The model under review builds one solid part; all positions refer to its coordinate system, in mm. A direction names the side the tool comes from. Give positions to 0.01 mm unless a question says otherwise; leave off trailing zeros. Loops run counter-clockwise (first coordinate to the right, second up) from the corner with the lowest first, then second, coordinate; pieces in that order, holes last. Notation, with made-up numbers: M 19,-22 L 50,-22 A11 cw 50,-3 Z; hole C 78,55.5 d3. An arc over 180 degrees is marked long. Put each result on its own line as item: value. Start each with the question number.
```python
from build123d import *

# Parameters (mm, degrees)
SKETCH1_W           = 50
SKETCH1_H           = 50
BOSS_EXTRUDE1_DEPTH = 2
SKETCH2_R           = 11
CUT_EXTRUDE1_DEPTH  = 36.411862419
CHAMFER1_SIZE       = 6
CHAMFER2_SIZE       = 6
CUT_EXTRUDE2_DEPTH  = 36.411862419
CIRPATTERN1_COUNT   = 4
SKETCH4_R           = 2
CUT_EXTRUDE3_DEPTH  = 36.411862419
SKETCH5_W           = 50
SKETCH5_H           = 2
BOSS_EXTRUDE5_DEPTH = 48
CHAMFER3_SIZE       = 6
CHAMFER4_SIZE       = 6
CUT_EXTRUDE5_DEPTH  = 74.681748079
BOSS_EXTRUDE6_START = -1
BOSS_EXTRUDE6_DEPTH = 1.000012
FILLET1_R           = 3


with BuildPart() as part:
    # Sketch1 → Boss-Extrude1 (new body)
    with BuildSketch(Plane.XY):
        Rectangle(SKETCH1_W, SKETCH1_H)
    extrude(amount=BOSS_EXTRUDE1_DEPTH)

    # Sketch2 → Cut-Extrude1 (cut, through all)
    with BuildSketch(Plane.XY.offset(2)):
        Circle(SKETCH2_R)
    extrude(amount=-CUT_EXTRUDE1_DEPTH, mode=Mode.SUBTRACT)

    # Chamfer1
    chamfer1_edges = [part.edges().sort_by_distance(p)[0] for p in [
        (-25, 25, 1),
    ]]
    chamfer(chamfer1_edges, length=CHAMFER1_SIZE)

    # Chamfer2
    chamfer2_edges = [part.edges().sort_by_distance(p)[0] for p in [
        (25, 25, 1),
    ]]
    chamfer(chamfer2_edges, length=CHAMFER2_SIZE)

    # Sketch3 → Cut-Extrude2 (cut, through all)
    with BuildSketch(Plane.XY.offset(2)):
        with BuildLine():
            Line((8.63247336, 12.016622274), (14.958263021, 16.914007818))
            ThreePointArc((14.958263021, 16.914007818), (17.764056822, 16.556906789), (17.406955793, 13.751112987))
            Line((17.406955793, 13.751112987), (11.081166132, 8.853727444))
            ThreePointArc((11.081166132, 8.853727444), (8.27537233, 9.210828473), (8.63247336, 12.016622274))
        make_face()
    cut_extrude2 = extrude(amount=-CUT_EXTRUDE2_DEPTH, mode=Mode.SUBTRACT)

    # CirPattern1: Cut-Extrude2 ×4 about axis
    cirpattern1_axis = Axis((0, 0, 0), (0, 0, 1))
    for i in range(1, CIRPATTERN1_COUNT):
        add(cut_extrude2.rotate(cirpattern1_axis, i * 360 / CIRPATTERN1_COUNT), mode=Mode.SUBTRACT)

    # Sketch4 → Cut-Extrude3 (cut, through all)
    with BuildSketch(Plane.XY.offset(2)):
        with Locations((14, 0)):
            Circle(SKETCH4_R)
    cut_extrude3 = extrude(amount=-CUT_EXTRUDE3_DEPTH, mode=Mode.SUBTRACT)

    # Mirror5: Cut-Extrude3 across plane
    add(cut_extrude3.mirror(Plane(origin=(0, 0, 0), x_dir=(0, 0, 1), z_dir=(1, 0, 0))), mode=Mode.SUBTRACT)

    # Sketch5 → Boss-Extrude5 (add)
    with BuildSketch(Plane(origin=(0, 0, 0), x_dir=(-1, 0, 0), z_dir=(0, 0, -1))):
        with Locations((0, -24)):
            Rectangle(SKETCH5_W, SKETCH5_H)
    extrude(amount=BOSS_EXTRUDE5_DEPTH)

    # Chamfer3
    chamfer3_edges = [part.edges().sort_by_distance(p)[0] for p in [
        (25, -24, -48),
    ]]
    chamfer(chamfer3_edges, length=CHAMFER3_SIZE)

    # Chamfer4
    chamfer4_edges = [part.edges().sort_by_distance(p)[0] for p in [
        (-25, -24, -48),
    ]]
    chamfer(chamfer4_edges, length=CHAMFER4_SIZE)

    # Sketch7 → Cut-Extrude5 (cut, through all)
    with BuildSketch(Plane.XZ.offset(25)):
        with BuildLine():
            Line((-13, -7.5), (-13, -36.5))
            ThreePointArc((-13, -36.5), (-15.5, -39), (-18, -36.5))
            Line((-18, -36.5), (-18, -7.5))
            ThreePointArc((-18, -7.5), (-15.5, -5), (-13, -7.5))
        make_face()
    cut_extrude5 = extrude(amount=-CUT_EXTRUDE5_DEPTH, mode=Mode.SUBTRACT)

    # Mirror8: Cut-Extrude5 across plane
    add(cut_extrude5.mirror(Plane(origin=(0, 0, 0), x_dir=(0, 0, 1), z_dir=(1, 0, 0))), mode=Mode.SUBTRACT)

    # Sketch8 → Boss-Extrude6 (add)
    with BuildSketch(Plane(origin=(25, 0, 0), x_dir=(0, 0, -1), z_dir=(1, 0, 0)).offset(BOSS_EXTRUDE6_START)):
        Polygon((0, -10.038318293), (9.843932034, -23), (0, -23), align=None)
    boss_extrude6 = extrude(amount=BOSS_EXTRUDE6_DEPTH)

    # Mirror9: Boss-Extrude6 across plane
    add(boss_extrude6.mirror(Plane(origin=(0, 0, 0), x_dir=(0, 0, 1), z_dir=(1, 0, 0))))

    # Fillet1
    fillet1_edges = [part.edges().sort_by_distance(p)[0] for p in [
        (0, -25, 2),
    ]]
    fillet(fillet1_edges, radius=FILLET1_R)


solid = part.part
```
Item 1: Draft analysis for pull direction X (two halves, no side actions). For faces 4 (the flat face through (0, -25, -24)), 5 (the cylindrical face through (15.6, -24, -5)), 6 (the flat face through (22, 22, 1)), 7 (the flat face through (-24, -19, -3)), state which applies: +X half, -X half, draft (parallel to the pull), parting line (faces both ways), or undercut.
Item 2: Tool access review of faces 1 (the cylindrical face through (0.35, -24.1, 1.14)), 2 (the flat face through (14.43, -11.75, 1.01)), 3 (the flat face through (0, 12, 0)): name each direction out of +Z, -Z, +X, -X, +Y, -Y from which nothing blocks a thin tool from reaching the whole face with its end or side.
Item 3: Consider section B-B, the plane y = 0. Write out the cut boundary in (x, z).
Item 4: To check wall thickness, follow L1, parallel to Y at x = -14, z = 0.65; L2, parallel to Y at x = -14, z = 1.55; L3, parallel to Z at x = -15, y = 21.5. State the ranges of each line that lie inside material, in increasing order. Write a range as [from, to].
Item 5: Consider section D-D, the plane x = 20. Write out the cut boundary in (y, z), plus the area to 3 significant figures.
Item 6: Clearance check with flat-ended pins moving along their axes: pin 1 Ø12 at (x, y) = (-14, 12) entering from -Z; pin 2 Ø20 at (x, y) = (0, 0) entering from -Z; pin 3 Ø1.5 at (x, z) = (7.5, -5.5) entering from +Y. State where each tip first meets the part, or that it passes through.
Item 7: Consider section A-A, the plane x = 0. Write out the cut boundary in (y, z), plus the area to 3 significant figures.
Item 8: Consider section C-C, the plane z = -18. Write out the cut boundary in (x, y), plus the area to 3 significant figures.
Report:
1. face 4: draft
1. face 5: undercut
1. face 6: +X half
1. face 7: undercut
2. face 1: +Z, +X, -X, -Y
2. face 2: +Z, -Z
2. face 3: -Z, +Y
3. outline: M -25,0 L -16,0 L -16,2 L -25,2 Z; M -12,0 L -11,0 L -11,2 L -12,2 Z; M 11,0 L 12,0 L 12,2 L 11,2 Z; M 16,0 L 25,0 L 25,2 L 16,2 Z
4. L1: [-24.51, -16.17], [-11.11, -2], [2, 11.19], [17.67, 25]
4. L2: [-23.58, -16.17], [-11.11, -2], [2, 11.19], [17.67, 25]
4. L3: [0, 2]
5. outline: M -25,-47 L -23,-47 L -23,0 L 24,0 L 24,2 L -22,2 A3 ccw -25,-1 Z
5. area: 190 mm²
6. pin 1: z = 0
6. pin 2: through
6. pin 3: y = -23
7. outline: M -25,-48 L -23,-48 L -23,0 L -11,0 L -11,2 L -22,2 A3 ccw -25,-1 Z; M 11,0 L 25,0 L 25,2 L 11,2 Z
7. area: 150 mm²
8. outline: M -25,-25 L -18,-25 L -18,-23 L -25,-23 Z; M -13,-25 L 13,-25 L 13,-23 L -13,-23 Z; M 18,-25 L 25,-25 L 25,-23 L 18,-23 Z
8. area: 80.0 mm²
